from build123d import *

# Parameters (mm, degrees)
F0_R     = 17.5
F0_R_2   = 14.5
F1_DEPTH = 10
F2_SIZE  = 0.75


with BuildPart() as f1:
    # F0 (on Right) → F1 (new body, symmetric)
    with BuildSketch(Plane.YZ):
        Circle(F0_R)
        Circle(F0_R_2, mode=Mode.SUBTRACT)
    extrude(amount=F1_DEPTH, both=True)

    # F2
    f2_edges = [f1.edges().sort_by_distance(p)[0] for p in [
        (-10, -17.5, 0),
        (10, -17.5, 0),
        (10, -14.5, 0),
        (-10, -14.5, 0),
    ]]
    chamfer(f2_edges, length=F2_SIZE)


solid = f1.part
Build history of the part. All positions in model axes, mm. Coordinates: 2 decimals unless noted, no trailing zeros. Order: outer loops, then holes, each group sorted by start corner. A loop starts at its lowest first (then second) coordinate and runs counter-clockwise, first axis right, second up. Notation, with made-up numbers: (51, 23.5) - (110, 23.5) arc R20 ccw to (110, 40.5) - close; hole circle Ø5 at (73.25, 10.5). An arc over 180 degrees is marked (long way). Write each question's results on one line, items separated by ' | '. Start each with the question number.
Item 1: Wall check: probe 1 along Z at (x, y) = (-0.75, 0); probe 2 along Y at (x, z) = (6.25, 0.5); probe 3 along Z at (x, y) = (2.5, 5). Give the ranges that are in metal, low to high. Write a range as [from, to].
Item 2: Flat gauge pins, fed straight in: pin 1 (1 mm diameter, centred on x = 6, z = 12, fed in from -Y); pin 2 (12 mm diameter, centred on y = 4, z = 0, fed in from -X); pin 3 (5 mm diameter, centred on x = 7.5, y = 6, fed in from -Z); pin 4 (1 mm diameter, centred on x = 2.5, y = 10, fed in from +Z). Where does each tip first touch, or does it go through?
Item 3: Mould opens along Y. For faces 1 (the face through (-0.13, 6.691, -12.864)), 2 (the face through (10, 4, -15)), 3 (the face through (0.13, -13.887, -10.648)) say: released by +Y, released by -Y, zero draft, split by the parting line, or undercut.
Item 4: Band-saw the part on A-A on z = 0. Write the cut outline in (x, y).
Item 5: Band-saw the part on C-C on x = 0. Write the cut outline in (y, z).
Numbers:
1) probe 1: [-17.5, -14.5], [14.5, 17.5] | probe 2: [-17.49, -14.49], [14.49, 17.49] | probe 3: [-16.77, -13.61], [13.61, 16.77]
2) pin 1: y = -13.19 | pin 2: through | pin 3: z = -17.15 | pin 4: z = 14.7
3) face 1: undercut | face 2: zero draft | face 3: split by the parting line
4) outline: (-10, -16.75) - (-9.25, -17.5) - (9.25, -17.5) - (10, -16.75) - (10, -15.25) - (9.25, -14.5) - (-9.25, -14.5) - (-10, -15.25) - close; (-10, 15.25) - (-9.25, 14.5) - (9.25, 14.5) - (10, 15.25) - (10, 16.75) - (9.25, 17.5) - (-9.25, 17.5) - (-10, 16.75) - close
5) outline: circle Ø35 at (0, 0); hole circle Ø29 at (0, 0)
